from build123d import *

# Parameters (mm, degrees)
TD_SKETCH_R                             = 0.79248
TL_FEATURE_DEPTH                        = 21.0312
TDF_STD_SKETCH_W                        = 2.09296
TDF_STD_SKETCH_H                        = 2.09296
TDF_STD_FEATURE_DEPTH                   = 22.061040395
ISA_20_STD_FEATURE_DEPTH                = 22.061040395
ISA_20_STD_FEATURE_DEPTH_BACK           = 22.061040395
VW_STD_FEATURE_DEPTH                    = 22.061040395
VW_STD_FEATURE_DEPTH_BACK               = 22.061040395
F_10BA_STD_FEATURE_DEPTH                = 22.061040503
F_10BA_STD_FEATURE_DEPTH_BACK           = 22.061040503
FRO_STD_FEATURE_DEPTH                   = 22.061040395
FRO_STD_FEATURE_DEPTH_BACK              = 22.061040395
C_STD_FEATURE_DEPTH                     = 22.061040395
C_STD_FEATURE_DEPTH_BACK                = 22.061040395
ERW_STD_FEATURE_DEPTH                   = 0.0254
H_STD_FEATURE_REACH                     = 22.896
H_STD_SKETCH_R                          = 0.01905
H_STD_SKETCH_3_R                        = 0.01905
FUNNEL_FINAL_DIAMETRE_STD_FEATURE_DEPTH = 2.499995
FUNNEL_FINAL_DIAMETRE_STD_FEATURE_DRAFT = -22.5
ROUND_BR_STD_FEATURE_START              = -1
ROUND_BR_STD_FEATURE_DEPTH              = 1.009339363
CBRA_STD_FEATURE_DEPTH                  = 0.00635


with BuildPart() as part:
    # TD_sketch → TL_feature (new body)
    with BuildSketch(Plane(origin=(0, 0, 0), x_dir=(1, 0, 0), z_dir=(0, 1, 0))):
        with Locations(Location((0, 0, 0), (0, 0, 270))):
            Circle(TD_SKETCH_R)
    extrude(amount=TL_FEATURE_DEPTH)

    # TDF_STD_sketch → TDF_STD_feature (cut, through all)
    with BuildSketch(Plane(origin=(0, 0, 0), x_dir=(1, 0, 0), z_dir=(0, 1, 0))):
        with Locations((-1.4224, 0)):
            Rectangle(TDF_STD_SKETCH_W, TDF_STD_SKETCH_H)
    extrude(amount=TDF_STD_FEATURE_DEPTH, mode=Mode.SUBTRACT)

    # ISA_20_STD_sketch → ISA_20_STD_feature (cut, two sides: drawn at the far end of the back side and taken through both)
    with BuildSketch(Plane(origin=(0, 0, 0), x_dir=(0, 0, -1), z_dir=(1, 0, 0)).offset(-ISA_20_STD_FEATURE_DEPTH_BACK)):
        Polygon((-12.955177728, 73.256388083), (-3.746467997, 21.0312), (-0.0381, 0), (0.0381, 0), (3.746467997, 21.0312), (12.955177728, 73.256388083), (12.955177728, -32.805303497), (-12.955177728, -32.805303497), align=None)
    extrude(amount=ISA_20_STD_FEATURE_DEPTH + ISA_20_STD_FEATURE_DEPTH_BACK, mode=Mode.SUBTRACT)

    # VW_STD_sketch → VW_STD_feature (cut, two sides: drawn at the far end of the back side and taken through both)
    with BuildSketch(Plane(origin=(0, 0, 0), x_dir=(0, 0, -1), z_dir=(1, 0, 0)).offset(-VW_STD_FEATURE_DEPTH_BACK)):
        with BuildLine():
            Line((-70.448918022, 70.704723144), (-20.775394878, 21.0312))
            Line((-20.775394878, 21.0312), (-0.087997439, 0.343802561))
            ThreePointArc((-0.087997439, 0.343802561), (-0.060467299, 0.302600796), (-0.0508, 0.254))
            Line((-0.0508, 0.254), (-0.0508, 0))
            Line((-0.0508, 0), (0.0508, 0))
            Line((0.0508, 0), (0.0508, 0.254))
            ThreePointArc((0.0508, 0.254), (0.060467299, 0.302600796), (0.087997439, 0.343802561))
            Line((0.087997439, 0.343802561), (20.775394878, 21.0312))
            Line((20.775394878, 21.0312), (70.448918022, 70.704723144))
            Line((70.448918022, 70.704723144), (70.448918022, -69.793217099))
            Line((70.448918022, -69.793217099), (-70.448918022, -69.793217099))
            Line((-70.448918022, -69.793217099), (-70.448918022, 70.704723144))
        make_face()
    extrude(amount=VW_STD_FEATURE_DEPTH + VW_STD_FEATURE_DEPTH_BACK, mode=Mode.SUBTRACT)

    # 10BA_STD_sketch → 10BA_STD_feature (cut, two sides: drawn at the far end of the back side and taken through both)
    with BuildSketch(Plane.XY.offset(-F_10BA_STD_FEATURE_DEPTH_BACK)):
        Polygon((-53.226091952, 0), (-0.37592, 0), (-0.25146, 0), (0.013312083, 0.046686462), (3.713447997, 21.0312), (12.890784046, 73.078459086), (91.272293968, 2.163710242), (25.155417971, -70.914748844), align=None)
    extrude(amount=F_10BA_STD_FEATURE_DEPTH + F_10BA_STD_FEATURE_DEPTH_BACK, mode=Mode.SUBTRACT)

    # FRO_STD_sketch → FRO_STD_feature (cut, two sides: drawn at the far end of the back side and taken through both)
    with BuildSketch(Plane.XY.offset(-FRO_STD_FEATURE_DEPTH_BACK)):
        with BuildLine():
            Line((-0.37592, 52.152138388), (-0.37592, 0.02794))
            ThreePointArc((-0.37592, 0.02794), (-0.367736563, 0.008183437), (-0.34798, 0))
            Line((-0.34798, 0), (51.776218388, 0))
            Line((51.776218388, 0), (-21.9385299, -73.714748288))
            Line((-21.9385299, -73.714748288), (-74.090668288, -21.5626099))
            Line((-74.090668288, -21.5626099), (-0.37592, 52.152138388))
        make_face()
    extrude(amount=FRO_STD_FEATURE_DEPTH + FRO_STD_FEATURE_DEPTH_BACK, mode=Mode.SUBTRACT)

    # C_STD_sketch → C_STD_feature (cut, two sides: drawn at the far end of the back side and taken through both)
    with BuildSketch(Plane(origin=(0, 0, 0), x_dir=(0, 0, -1), z_dir=(1, 0, 0)).offset(-C_STD_FEATURE_DEPTH_BACK)):
        with BuildLine():
            Line((-50.8957695, -11.2378876), (-0.027944581, 0))
            ThreePointArc((-0.027944581, 0), (0, 0.003050032), (0.027944581, 0))
            Line((0.027944581, 0), (50.8957695, -11.2378876))
            Line((50.8957695, -11.2378876), (50.8957695, -115.426672595))
            Line((50.8957695, -115.426672595), (-50.8957695, -115.426672595))
            Line((-50.8957695, -115.426672595), (-50.8957695, -11.2378876))
        make_face()
    extrude(amount=C_STD_FEATURE_DEPTH + C_STD_FEATURE_DEPTH_BACK, mode=Mode.SUBTRACT)


with BuildPart() as body_2:
    # ERW_STD_sketch → ERW_STD_feature (new, symmetric)
    with BuildSketch(Plane.XY):
        Polygon((-0.1397, 0.09144), (-0.1397, 0), (-0.32512, 0), (-0.272327091, 0.09144), align=None)
    extrude(amount=ERW_STD_FEATURE_DEPTH, both=True)

    # H_STD_sketch → H_STD_feature (add, up to next)
    with BuildSketch(Plane(origin=(-0.010357492, 0.166115932, 0), x_dir=(0, 0, -1), z_dir=(0.8660254037844415, 0.4999999999999953, 0)), mode=Mode.PRIVATE) as h_std_feature_sk1:
        with Locations(Location((0, 0, 0), (0, 0, 90))):
            Circle(H_STD_SKETCH_R)
    h_std_feature_tool1 = extrude(h_std_feature_sk1.sketch, amount=-H_STD_FEATURE_REACH, mode=Mode.PRIVATE) - body_2.part
    add(h_std_feature_tool1.solids().sort_by_distance((-0.010357, 0.166116, 0))[0])


with BuildPart() as funnel_final_diametre_std_feature_tool:
    # H_STD_sketch<3> → funnel_final_diametre_STD_feature (with draft: the straight prism first)
    with BuildSketch(Plane(origin=(-0.010357492, 0.166115932, 0), x_dir=(0, 0, -1), z_dir=(0.8660254037844415, 0.4999999999999953, 0))):
        with Locations(Location((0, 0, 0), (0, 0, 90))):
            Circle(H_STD_SKETCH_3_R)
    extrude(amount=FUNNEL_FINAL_DIAMETRE_STD_FEATURE_DEPTH)
    # funnel_final_diametre_STD_feature: the draft: its side faces are tilted about the plane it starts from
    funnel_final_diametre_std_feature_sides = [funnel_final_diametre_std_feature_tool.faces().sort_by_distance(p)[0] for p in [
        (1.081697098, 0.774616898, 0),
    ]]
    draft(funnel_final_diametre_std_feature_sides, Plane(origin=(-0.010357492, 0.166115932, 0), x_dir=(0, 0, -1), z_dir=(0.8660254037844415, 0.4999999999999953, 0)), FUNNEL_FINAL_DIAMETRE_STD_FEATURE_DRAFT)


with BuildPart() as body_2_1:
    add(body_2.part)

    # funnel_final_diametre_STD_feature: add funnel_final_diametre_std_feature_tool
    add(funnel_final_diametre_std_feature_tool.part)

    # ROUND_BR_STD_feature: read off the stored shape, not the designer's step
    # ROUND_BR_STD_feature outline → ROUND_BR_STD_feature (cut)
    with BuildSketch(Plane(origin=(0, 0, 0), x_dir=(0.8660254037844362, -0.5000000000000042, 0), z_dir=(0.5000000000000042, 0.8660254037844363, 0)).offset(ROUND_BR_STD_FEATURE_START)):
        with BuildLine():
            Line((-0.281562179, -0.0254), (-0.256162179, -0.0254))
            ThreePointArc((-0.256162179, -0.0254), (-0.274122691, -0.017960512), (-0.281562179, 0))
            Line((-0.281562179, 0), (-0.281562179, -0.0254))
        make_face()
        with BuildLine():
            Line((-0.281562179, 0.0254), (-0.281562179, 0))
            ThreePointArc((-0.281562179, 0), (-0.274122691, 0.017960512), (-0.256162179, 0.0254))
            Line((-0.256162179, 0.0254), (-0.281562179, 0.0254))
        make_face()
    extrude(amount=ROUND_BR_STD_FEATURE_DEPTH, mode=Mode.SUBTRACT)


with BuildPart() as part_1:
    add(part.part)

    # COMBINE_STD_feature: cut body 2
    add(body_2_1.part, mode=Mode.SUBTRACT)

    # CBRA_STD_sketch → CBRA_STD_feature (cut, symmetric)
    with BuildSketch(Plane.XY):
        Polygon((-0.319782487, 0.009244844), (-0.345182487, 0), (-0.319782487, 0), align=None)
    extrude(amount=CBRA_STD_FEATURE_DEPTH, both=True, mode=Mode.SUBTRACT)


solid = part_1.part
Here's how the part is built. I have some questions about the finished solid (model axes, mm). Round coordinates to 2 decimals unless told otherwise and drop trailing zeros. Loops run counter-clockwise (first coordinate to the right, second up) from the corner with the lowest first, then second, coordinate; pieces in that order, holes last. Notation, with made-up numbers: M 48,25.5 L 85,25.5 A30 cw 85,60.5 Z; hole C -3.5,-3 d6. An arc over 180 degrees is marked long. Write each question's results on one line, items separated by ' | '. Start each with the question number.
(1) If I drill on probe 1 along X at (y, z) = (18.75, -0.05); probe 2 along Z at (x, y) = (0.3, 9.5); probe 3 along X at (y, z) = (15.75, -0.6), over which ranges is the centre line in solid material (lowest first)? Write a range as from..to.
(2) I want a section at B-B (y = 13). Please give me the cut outline in (x, z).
(3) I want a section at C-C (x = 0.25). Please give me the cut outline in (y, z), then the cut area to 3 significant figures.
(4) I want a section at A-A (z = 0.3). Please give me the cut outline in (x, y), then the cut area to 3 significant figures.
Solved:
1) probe 1: x = -0.38..0.79 | probe 2: z = -0.73..0.73 | probe 3: x = -0.38..0.52
2) outline: M -0.38,-0.7 A0.79 ccw long -0.38,0.7 Z
3) outline: M 1.39,-0.28 L 4.05,-0.75 L 21.03,-0.75 L 21.03,0.75 L 4.05,0.75 L 1.39,0.28 Z | area: 28.3 mm²
4) outline: M -0.38,1.49 L 0.27,1.49 L 0.73,4.13 L 0.73,21.03 L -0.38,21.03 Z | area: 21.1 mm²
